Input: part model. Units: mm. Frame: model coordinates. A direction names the side the tool comes from. Coordinates: 2 decimals unless noted, no trailing zeros. Order: outer loops, then holes, each group sorted by start corner. A loop starts at its lowest first (then second) coordinate and runs counter-clockwise, first axis right, second up. Notation, with made-up numbers: (-17.5, -31.5) -> (3.5, -31.5) arc R17 cw to (3.5, -23.5) -> close; hole circle Ø7 at (29, 45.25). An arc over 180 degrees is marked (long way). One line per question, with ' | ' between items.
```python
from build123d import *

# Parameters (mm, degrees)
SCHIZZO1_R                   = 2.5
SCHIZZO1_R_2                 = 2.05
ESTRUSIONE_ESTRUSIONE1_DEPTH = 5
SCHIZZO2_R                   = 2.05
TAGLIO_ESTRUSIONE1_DEPTH     = 6
CROQUIS1_W                   = 24.155603231
CROQUIS1_H                   = 18.627416998
CORTAR_EXTRUIR1_DEPTH        = 10
FILLET1_R                    = 5
CUT_EXTRUDE1_REACH           = 7
SKETCH1_R                    = 2.899137803
CUT_EXTRUDE2_REACH           = 7
SKETCH2_R                    = 2.05


with BuildPart() as part:
    # Schizzo1 → Estrusione-Estrusione1 (new body)
    with BuildSketch(Plane.XY):
        with BuildLine():
            Line((39.155603231, -41.372583002), (-35, -41.372583002))
            Line((-35, -41.372583002), (-35, -31.372583002))
            Line((-35, -31.372583002), (-47.627416998, -31.372583002))
            Line((-47.627416998, -31.372583002), (-47.627416998, 18.627416998))
            Line((-47.627416998, 18.627416998), (-27.627416998, 18.627416998))
            Line((-27.627416998, 18.627416998), (-27.627416998, 22.627416998))
            ThreePointArc((-27.627416998, 22.627416998), (-26.162950904, 26.162950904), (-22.627416998, 27.627416998))
            Line((-22.627416998, 27.627416998), (19.155603231, 27.627416998))
            ThreePointArc((19.155603231, 27.627416998), (33.297738855, 21.769552622), (39.155603231, 7.627416998))
            Line((39.155603231, 7.627416998), (39.155603231, -41.372583002))
        make_face()
        Circle(SCHIZZO1_R, mode=Mode.SUBTRACT)
        with Locations((-20, -38.872583002)):
            Circle(SCHIZZO1_R_2, mode=Mode.SUBTRACT)
        with Locations((0, -38.872583002)):
            Circle(SCHIZZO1_R_2, mode=Mode.SUBTRACT)
        with Locations((-22.627416998, 22.627416998)):
            Circle(SCHIZZO1_R_2, mode=Mode.SUBTRACT)
    extrude(amount=ESTRUSIONE_ESTRUSIONE1_DEPTH)

    # Schizzo2 → Taglio-Estrusione1 (cut, through all)
    with BuildSketch(Plane.XY.offset(5)):
        with Locations((-17.707593382, -6.797308246)):
            Circle(SCHIZZO2_R)
        with Locations((8.435926092, 3.238248629)):
            Circle(SCHIZZO2_R)
        Polygon((-12.894665672, -11.698011855), (8.138901337, -3.623981952), (3.623465173, 8.139131422), (-17.410101836, 0.065101519), align=None)
    extrude(amount=-TAGLIO_ESTRUSIONE1_DEPTH, mode=Mode.SUBTRACT)

    # Croquis1 → Cortar-Extruir1 (cut)
    with BuildSketch(Plane(origin=(0, 0, 0), x_dir=(-1, 0, 0), z_dir=(0, 0, -1))):
        with Locations((-27.077801616, -40.686291501)):
            Rectangle(CROQUIS1_W, CROQUIS1_H)
    extrude(amount=-CORTAR_EXTRUIR1_DEPTH, mode=Mode.SUBTRACT)

    # Fillet1
    fillet1_edges = [part.edges().sort_by_distance(p)[0] for p in [
        (-47.627416998, 18.627416998, 2.5),
    ]]
    fillet(fillet1_edges, radius=FILLET1_R)

    # Sketch1 → Cut-Extrude1 (cut, up to next)
    with BuildSketch(Plane.XY.offset(5), mode=Mode.PRIVATE) as cut_extrude1_sk1:
        with Locations((-35, -31.372583002)):
            Circle(SKETCH1_R)
    cut_extrude1_tool1 = extrude(cut_extrude1_sk1.sketch, amount=-CUT_EXTRUDE1_REACH, mode=Mode.PRIVATE) & part.part
    add(cut_extrude1_tool1.solids().sort_by_distance((-35, -31.372583, 5))[0], mode=Mode.SUBTRACT)
    # Sketch1 → Cut-Extrude1 (cut, up to next)
    with BuildSketch(Plane.XY.offset(5), mode=Mode.PRIVATE) as cut_extrude1_sk2:
        with Locations((15, -31.372583002)):
            Circle(SKETCH1_R)
    cut_extrude1_tool2 = extrude(cut_extrude1_sk2.sketch, amount=-CUT_EXTRUDE1_REACH, mode=Mode.PRIVATE) & part.part
    add(cut_extrude1_tool2.solids().sort_by_distance((15, -31.372583, 5))[0], mode=Mode.SUBTRACT)
    # Sketch1 → Cut-Extrude1 (cut, up to next)
    with BuildSketch(Plane.XY.offset(5), mode=Mode.PRIVATE) as cut_extrude1_sk3:
        with BuildLine():
            Line((-17.95, -38.872583002), (-17.95, -41.372583002))
            ThreePointArc((-17.95, -41.372583002), (-20, -43.422583002), (-22.05, -41.372583002))
            Line((-22.05, -41.372583002), (-22.05, -38.872583002))
            ThreePointArc((-22.05, -38.872583002), (-20, -36.822583002), (-17.95, -38.872583002))
        make_face()
    cut_extrude1_tool3 = extrude(cut_extrude1_sk3.sketch, amount=-CUT_EXTRUDE1_REACH, mode=Mode.PRIVATE) & part.part
    add(cut_extrude1_tool3.solids().sort_by_distance((-20, -40.122583, 5))[0], mode=Mode.SUBTRACT)
    # Sketch1 → Cut-Extrude1 (cut, up to next)
    with BuildSketch(Plane.XY.offset(5), mode=Mode.PRIVATE) as cut_extrude1_sk4:
        with BuildLine():
            Line((2.05, -38.872583002), (2.05, -41.372583002))
            ThreePointArc((2.05, -41.372583002), (0, -43.422583002), (-2.05, -41.372583002))
            Line((-2.05, -41.372583002), (-2.05, -38.872583002))
            ThreePointArc((-2.05, -38.872583002), (0, -36.822583002), (2.05, -38.872583002))
        make_face()
    cut_extrude1_tool4 = extrude(cut_extrude1_sk4.sketch, amount=-CUT_EXTRUDE1_REACH, mode=Mode.PRIVATE) & part.part
    add(cut_extrude1_tool4.solids().sort_by_distance((0, -40.122583, 5))[0], mode=Mode.SUBTRACT)

    # Sketch2 → Cut-Extrude2 (cut, up to next)
    with BuildSketch(Plane.XY.offset(5), mode=Mode.PRIVATE) as cut_extrude2_sk1:
        with Locations((-12.894665672, -11.698011855)):
            Circle(SKETCH2_R)
    cut_extrude2_tool1 = extrude(cut_extrude2_sk1.sketch, amount=-CUT_EXTRUDE2_REACH, mode=Mode.PRIVATE) & part.part
    add(cut_extrude2_tool1.solids().sort_by_distance((-12.894666, -11.698012, 5))[0], mode=Mode.SUBTRACT)
    # Sketch2 → Cut-Extrude2 (cut, up to next)
    with BuildSketch(Plane.XY.offset(5), mode=Mode.PRIVATE) as cut_extrude2_sk2:
        with Locations((8.138901337, -3.623981952)):
            Circle(SKETCH2_R)
    cut_extrude2_tool2 = extrude(cut_extrude2_sk2.sketch, amount=-CUT_EXTRUDE2_REACH, mode=Mode.PRIVATE) & part.part
    add(cut_extrude2_tool2.solids().sort_by_distance((8.138901, -3.623982, 5))[0], mode=Mode.SUBTRACT)
    # Sketch2 → Cut-Extrude2 (cut, up to next)
    with BuildSketch(Plane.XY.offset(5), mode=Mode.PRIVATE) as cut_extrude2_sk3:
        with Locations((3.623465173, 8.139131422)):
            Circle(SKETCH2_R)
    cut_extrude2_tool3 = extrude(cut_extrude2_sk3.sketch, amount=-CUT_EXTRUDE2_REACH, mode=Mode.PRIVATE) & part.part
    add(cut_extrude2_tool3.solids().sort_by_distance((3.623465, 8.139131, 5))[0], mode=Mode.SUBTRACT)
    # Sketch2 → Cut-Extrude2 (cut, up to next)
    with BuildSketch(Plane.XY.offset(5), mode=Mode.PRIVATE) as cut_extrude2_sk4:
        with Locations((-17.410101836, 0.065101519)):
            Circle(SKETCH2_R)
    cut_extrude2_tool4 = extrude(cut_extrude2_sk4.sketch, amount=-CUT_EXTRUDE2_REACH, mode=Mode.PRIVATE) & part.part
    add(cut_extrude2_tool4.solids().sort_by_distance((-17.410102, 0.065102, 5))[0], mode=Mode.SUBTRACT)


solid = part.part
```
1. Cut plane B-B, the plane x = 14. Return loops of the section in (y, z), and give its area (3 significant figures).
Recorded:
outline: (-41.37, 0) -> (-34.09, 0) -> (-34.09, 5) -> (-41.37, 5) -> close; (-28.65, 0) -> (27.63, 0) -> (27.63, 5) -> (-28.65, 5) -> close | area: 318 mm^2
2. Ray query, line 1 (X direction, y = 23.5, z = 3.65); line 2 (Y direction, x = 8, z = 1.45); line 3 (X direction, y = 8.5, z = 1.7). Return the intervals inside material, ascending. Write a range as [from, to].
Recorded:
line 1: x = [-27.55, -24.48], [-20.77, 31.32] | line 2: y = [-41.37, -5.67], [-1.58, 1.24], [5.24, 27.63] | line 3: x = [-47.63, 1.61], [5.64, 39.14]
3. Access query for faces 1 (the face through (-2.5, -7.71, 2.54)), 2 (the face through (-17.95, -40, 3)), 3 (the face through (-46.124, 17.202, 2.535)). Directions: +Z, -Z, +X, -X, +Y, -Y. A direction counts if a zero-diameter tool reaches every point of the face in a straight line with its end or side. Return the directions, or none.
Recorded:
face 1: +Z, -Z | face 2: +Z, -Z, -Y | face 3: +Z, -Z, -X, +Y
4. Cut plane C-C, the plane x = 0. Return loops of the section in (y, z), and give its area (3 significant figures).
Recorded:
outline: (-36.82, 0) -> (-6.75, 0) -> (-6.75, 5) -> (-36.82, 5) -> close; (6.75, 0) -> (27.63, 0) -> (27.63, 5) -> (6.75, 5) -> close | area: 255 mm^2
5. Mould query, pull axis X, two halves, no side actions, for faces 4 (the face through (-27.627, 21, 2)), 5 (the face through (39.156, -12, 2)), 6 (the face through (7.992, 1.237, 2.535)), 7 (the face through (29, -31.373, 2)). Classes: released by +X, released by -X, zero draft, split by the parting line, or undercut.
Recorded:
face 4: released by -X | face 5: released by +X | face 6: undercut | face 7: zero draft
6. Pin query (flat end, axial travel): pin 1 Ø3 at (y, z) = (21, 2) entering from -X; pin 2 Ø2 at (y, z) = (-39.5, 2.5) entering from +X; pin 3 Ø6.5 at (x, y) = (8.44, 3.24) entering from +Z; pin 4 Ø2.5 at (y, z) = (-38, 2.5) entering from -X. Return the tip coordinate at first contact, or that it passes through.
Recorded:
pin 1: stops at x = -27.63 | pin 2: stops at x = 15 | pin 3: stops at z = 5 | pin 4: stops at x = -35
7. Cut plane A-A, the plane z = 2.8. State how many separate pieces and enclosed holes the cut face has, and give its area (3 significant figures).
Recorded:
separate pieces: 1 | enclosed holes: 4 | area: 4,910 mm^2
8. Cut plane D-D, the plane x = 34. Return loops of the section in (y, z).
Recorded:
outline: (-31.37, 0) -> (21.03, 0) -> (21.03, 5) -> (-31.37, 5) -> close
